Autodesk Inventor part; units mm, degrees
ref_plane "YZ Plane" through (0, 0, 0) normal (1, 0, 0) x (0, 1, 0)
ref_plane "XZ Plane" through (0, 0, 0) normal (0, 1, 0) x (-1, 0, 0)
ref_plane "XY Plane" through (0, 0, 0) normal (0, 0, 1) x (1, 0, 0)
sketch "Sketch1" plane through (0, 0, 0) normal (1, 0, 0) x (0, 1, 0)
  line L0 (-6.35, -1.9593) -> (-6.35, 1.9593)
  line L1 (-4.8718, 4.5196) -> (-1.4782, 6.4789)
  line L2 (1.4782, 6.4789) -> (4.8718, 4.5196)
  line L3 (6.35, 1.9593) -> (6.35, -1.9593)
  line L4 (4.8718, -4.5196) -> (1.4782, -6.4789)
  line L5 (-1.4782, -6.4789) -> (-4.8718, -4.5196)
  arc A0 (4.8718, -4.5196) -> (6.35, -1.9593) centre (3.3937, -1.9593) ccw
  arc A1 (-1.4782, -6.4789) -> (1.4782, -6.4789) centre (0, -3.9187) ccw
  arc A2 (-6.35, -1.9593) -> (-4.8718, -4.5196) centre (-3.3937, -1.9593) ccw
  arc A3 (-4.8718, 4.5196) -> (-6.35, 1.9593) centre (-3.3937, 1.9593) ccw
  arc A4 (1.4782, 6.4789) -> (-1.4782, 6.4789) centre (0, 3.9187) ccw
  arc A5 (6.35, 1.9593) -> (4.8718, 4.5196) centre (3.3937, 1.9593) ccw
  circle A6 centre (0, 0) radius 6.875 construction
  point P0 (-6.35, -3.6662)
  point P1 (-6.35, 3.6662)
  point P2 (0, 7.3323)
  point P3 (6.35, 3.6662)
  point P4 (6.35, -3.6662)
  point P5 (0, -7.3323)
  dimension "d1" = 12.7
  dimension "d2" = 13.75
extrude "Extrusion1" add sketch "Sketch1" along normal blind 198.0875
sketch "Sketch2" plane through (0, 0, 0) normal (-1, 0, 0) x (0, 0, 1)
  point P0 (0, 0)
  point P1 (0, 0)
hole "Hole1" at (0, 0, 0) direction (1, 0, 0) diameter 3.9624 end through all
properties part number "STOCK,HEX,ROUND,HOOD" material "Aluminum 6061"
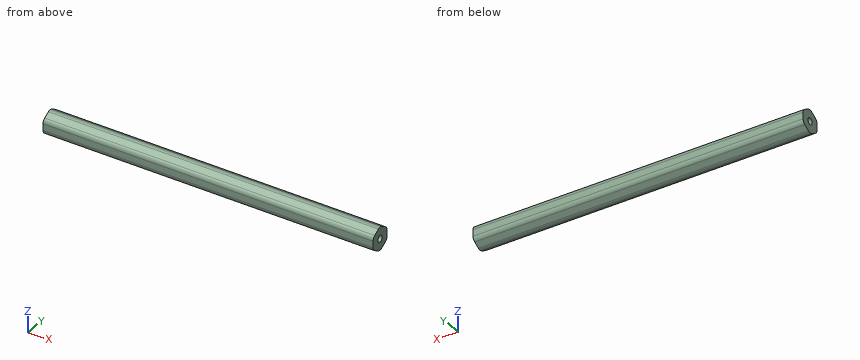
CAD build for the part. Positions are in the model's coordinates, mm. Coordinates: 2 decimals unless noted, no trailing zeros. Order: outer loops, then holes, each group sorted by start corner. A loop starts at its lowest first (then second) coordinate and runs counter-clockwise, first axis right, second up.
Item 1: Pin check, flat tips, straight feed: pin 1 Ø2 at (x, y) = (114.5, -4) entering from -Z; pin 2 Ø3 at (x, y) = (112.5, -5) entering from +Z. Stop position of each tip, or through.
Check sheet entries:
pin 1: stops at z = -5.6
pin 2: stops at z = 5.31
Item 2: Band-saw the part on A-A on x = 114. List the corners of the cut face in (y, z).
Check sheet entries:
outline: (-6.35, -1.96) arc R2.96 ccw to (-4.87, -4.52) - (-1.48, -6.48) arc R2.96 ccw to (1.48, -6.48) - (4.87, -4.52) arc R2.96 ccw to (6.35, -1.96) - (6.35, 1.96) arc R2.96 ccw to (4.87, 4.52) - (1.48, 6.48) arc R2.96 ccw to (-1.48, 6.48) - (-4.87, 4.52) arc R2.96 ccw to (-6.35, 1.96) - close; hole circle Ø3.96 at (0, 0)
Item 3: Band-saw the part on B-B on z = 0. List the corners of the cut face in (x, y), plus the area to 3 significant figures.
Check sheet entries:
outline: (0, -6.35) - (198.09, -6.35) - (198.09, -1.98) - (0, -1.98) - close; (0, 1.98) - (198.09, 1.98) - (198.09, 6.35) - (0, 6.35) - close
area: 1,730 mm2
Item 4: Drill centre lines: L1, parallel to Z at x = 158.5, y = 0 (3 decimals); L2, parallel to Y at x = 82, z = 0; L3, parallel to Z at x = 76, y = 1.5. Where is each one in solid material? Low to high.
Check sheet entries:
L1: z = -6.875 to -1.981, 1.981 to 6.875
L2: y = -6.35 to -1.98, 1.98 to 6.35
L3: z = -6.47 to -1.29, 1.29 to 6.47
